CAD build for the part. Positions are in the model's coordinates, mm. A direction names the side the tool comes from. Round coordinates to 2 decimals unless told otherwise and drop trailing zeros. Order: outer loops, then holes, each group sorted by start corner. A loop starts at its lowest first (then second) coordinate and runs counter-clockwise, first axis right, second up. Notation, with made-up numbers: (60, 68.5) -> (70, 68.5) arc R22 cw to (70, 81.5) -> close; hole circle Ø5 at (14, 59). An arc over 180 degrees is marked (long way). Return JSON: item names as keys, results as strings. Group by question number.
Q1. Cut at C-C (z = -46.5). Write the cut outline in (x, y), then the cut area to 3 significant figures.
Q2. Probe line 1 along Z through (x, y) = (-1, 6.5); line 2 along Z through (x, y) = (3.5, 48); line 3 along X through (y, z) = (11.5, 10). List the from-to ranges inside material, lowest first.
Q3. Cut at B-B (x = 0). Write the cut outline in (y, z), then the cut area to 3 significant figures.
Q4. Cut at A-A (y = 43). Write the cut outline in (x, z), then the cut area to 3 significant figures.
Q5. Cut at D-D (x = -42.5). Write the cut outline in (y, z).
Q6. Mould opens along Y. For faces 1 (the flat face through (18, 52, 8)), 2 (the cylindrical face through (-19.6, 50.99, 7.53)), 3 (the flat face through (1, 0, -1)), 4 (the flat face through (0.286, 30.097, -1.2)) say: +Y half, -Y half, draft (parallel to the pull), parting line (faces both ways), or undercut.
Q7. Flat gauge pins, fed straight in: pin 1 (10 mm diameter, centred on x = 59, y = 9, fed in from -Z); pin 2 (25 mm diameter, centred on x = 0, z = 8, fed in from -Y); pin 3 (4 mm diameter, centred on x = 58.5, z = 20, fed in from +Y); pin 4 (12 mm diameter, centred on y = 45, z = -37, fed in from +X). Where does each tip first touch, or does it go through?
Q8. Which spindle directions (+Z, -Z, +X, -X, +Y, -Y) get a long thin tool onto all of the face, cutting with end or side? Do faces 5 (the flat face through (-17, 52, 8)), 6 (the flat face through (10.21, 40.27, 22.21)), 7 (the flat face through (0, 15, 3.182)). Say none if no direction does.
from build123d import *

# Parameters (mm, degrees)
SKETCH1_R               = 75
BOSS_EXTRUDE1_DEPTH     = 50
SHELL1_T                = -5
SKETCH2_R               = 21
BOSS_EXTRUDE2_DEPTH     = 45
CUT_EXTRUDE1_START      = -19.2
CUT_EXTRUDE1_DEPTH      = 19.2
SKETCH3_3_R             = 2.15
BOSS_EXTRUDE3_DEPTH     = 2
CUT_EXTRUDE3_DEPTH      = 32
CUT_EXTRUDE3_DEPTH_BACK = 27


with BuildPart() as part:
    # Sketch1 → Boss-Extrude1 (new body)
    with BuildSketch(Plane(origin=(0, 0, 0), x_dir=(1, 0, 0), z_dir=(0, 1, 0))):
        with Locations(Location((0, 0, 0), (0, 0, 270))):
            Circle(SKETCH1_R)
    extrude(amount=BOSS_EXTRUDE1_DEPTH)

    # Shell1
    shell1_openings = [part.faces().sort_by_distance(p)[0] for p in [
        (0, 50, 0),
    ]]
    offset(amount=SHELL1_T, openings=shell1_openings, kind=Kind.INTERSECTION)

    # Sketch2 → Boss-Extrude2 (add)
    with BuildSketch(Plane(origin=(0, 5, 0), x_dir=(1, 0, 0), z_dir=(0, 1, 0))):
        with Locations(Location((0, -8, 0), (0, 0, 270))):
            Circle(SKETCH2_R)
    extrude(amount=BOSS_EXTRUDE2_DEPTH)

    # Sketch3 → Cut-Extrude1 (cut)
    with BuildSketch(Plane(origin=(0, 50, 0), x_dir=(1, 0, 0), z_dir=(0, 1, 0)).offset(CUT_EXTRUDE1_START)):
        with BuildLine():
            Line((11.193269132, -25.768250508), (9.2, -18.552724767))
            ThreePointArc((9.2, -18.552724767), (0, 6), (-9.2, -18.552724767))
            Line((-9.2, -18.552724767), (-11.193269132, -25.768250508))
            ThreePointArc((-11.193269132, -25.768250508), (0, -29), (11.193269132, -25.768250508))
        make_face()
    extrude(amount=CUT_EXTRUDE1_DEPTH, mode=Mode.SUBTRACT)

    # Sketch3<3> → Boss-Extrude3 (add)
    with BuildSketch(Plane(origin=(0, 50, 0), x_dir=(1, 0, 0), z_dir=(0, 1, 0))):
        with Locations(Location((-17.5, -8, 0), (0, 0, 270))):
            Circle(SKETCH3_3_R)
        with Locations(Location((17.5, -8, 0), (0, 0, 270))):
            Circle(SKETCH3_3_R)
    extrude(amount=BOSS_EXTRUDE3_DEPTH)

    # Sketch6 → Cut-Extrude3 (cut, two sides: drawn at the far end of the back side and taken through both)
    with BuildSketch(Plane(origin=(0, 50, -13), x_dir=(0, 0, 1), z_dir=(-1, 0, 0)).offset(-CUT_EXTRUDE3_DEPTH_BACK)):
        Polygon((-3.408673703, -45), (16.182064941, -45), (16.182064941, -23.856535334), (0, -9.257667594), (-3.408673703, -9.257667594), align=None)
    extrude(amount=CUT_EXTRUDE3_DEPTH + CUT_EXTRUDE3_DEPTH_BACK, mode=Mode.SUBTRACT)


solid = part.part
Solution:
{
 "1": {"outline": "(-58.85, 0) -> (58.85, 0) -> (58.85, 50) -> (52.32, 50) -> (52.32, 5) -> (-52.32, 5) -> (-52.32, 50) -> (-58.85, 50) -> close", "area": "1,180 mm²"},
 "2": {"line 1": "z = -74.99 to -69.99, 3.18 to 28.98, 69.99 to 74.99", "line 2": "z = -74.92 to -69.91, -12.71 to -5.56, 69.91 to 74.92", "line 3": "x = -74.33 to -69.28, -20.9 to 20.9, 69.28 to 74.33"},
 "3": {"outline": "(0, -75) -> (50, -75) -> (50, -70) -> (5, -70) -> (5, 3.18) -> (26.14, 3.18) -> (30.8, -1.98) -> (30.8, 29) -> (5, 29) -> (5, 70) -> (50, 70) -> (50, 75) -> (0, 75) -> close; (34.43, -6) -> (40.74, -13) -> (50, -13) -> (50, -6) -> close", "area": "1,970 mm²"},
 "4": {"outline": "circle Ø150 at (0, 0); (-11.19, 25.77) arc R21 ccw (long way) to (11.19, 25.77) -> (9.2, 18.55) arc R14 cw (long way) to (-9.2, 18.55) -> close; hole circle Ø140 at (0, 0)", "area": "2,890 mm²"},
 "5": {"outline": "(0, -61.8) -> (50, -61.8) -> (50, -55.62) -> (5, -55.62) -> (5, 55.62) -> (50, 55.62) -> (50, 61.8) -> (0, 61.8) -> close"},
 "6": {"face 1": "+Y half", "face 2": "draft", "face 3": "-Y half", "face 4": "undercut"},
 "7": {"pin 1": "stops at z = -52.05", "pin 2": "stops at y = 0", "pin 3": "stops at y = 5", "pin 4": "stops at x = 68.29"},
 "8": {"face 5": "+Z, -Z, +X, -X, +Y", "face 6": "+Y", "face 7": "none"}
}
